```python
from build123d import *

# Parameters (mm, degrees)
SKETCH1_W           = 4.6
SKETCH1_H           = 4.6
BOSS_EXTRUDE1_DEPTH = 50


with BuildPart() as part:
    # Sketch1 → Boss-Extrude1 (new body, symmetric)
    with BuildSketch(Plane.XY):
        with BuildLine():
            Line((15, -13), (15, -4.4))
            ThreePointArc((15, -4.4), (14.853553391, -4.046446609), (14.5, -3.9))
            Line((14.5, -3.9), (13.5, -3.9))
            ThreePointArc((13.5, -3.9), (13.146446609, -4.046446609), (13, -4.4))
            Line((13, -4.4), (13, -6.6))
            ThreePointArc((13, -6.6), (12.853553391, -6.953553391), (12.5, -7.1))
            Line((12.5, -7.1), (8.297056275, -7.1))
            ThreePointArc((8.297056275, -7.1), (8.105714559, -7.061939766), (7.943502884, -6.953553391))
            Line((7.943502884, -6.953553391), (6.096446609, -5.106497116))
            ThreePointArc((6.096446609, -5.106497116), (5.988060234, -4.944285441), (5.95, -4.752943725))
            Line((5.95, -4.752943725), (5.95, 4.752943725))
            ThreePointArc((5.95, 4.752943725), (5.988060234, 4.944285441), (6.096446609, 5.106497116))
            Line((6.096446609, 5.106497116), (7.943502884, 6.953553391))
            ThreePointArc((7.943502884, 6.953553391), (8.105714559, 7.061939766), (8.297056275, 7.1))
            Line((8.297056275, 7.1), (12.5, 7.1))
            ThreePointArc((12.5, 7.1), (12.853553391, 6.953553391), (13, 6.6))
            Line((13, 6.6), (13, 4.4))
            ThreePointArc((13, 4.4), (13.146446609, 4.046446609), (13.5, 3.9))
            Line((13.5, 3.9), (14.5, 3.9))
            ThreePointArc((14.5, 3.9), (14.853553391, 4.046446609), (15, 4.4))
            Line((15, 4.4), (15, 13))
            ThreePointArc((15, 13), (14.414213562, 14.414213562), (13, 15))
            Line((13, 15), (4.4, 15))
            ThreePointArc((4.4, 15), (4.046446609, 14.853553391), (3.9, 14.5))
            Line((3.9, 14.5), (3.9, 13.5))
            ThreePointArc((3.9, 13.5), (4.046446609, 13.146446609), (4.4, 13))
            Line((4.4, 13), (6.6, 13))
            ThreePointArc((6.6, 13), (6.953553391, 12.853553391), (7.1, 12.5))
            Line((7.1, 12.5), (7.1, 8.297056275))
            ThreePointArc((7.1, 8.297056275), (7.061939766, 8.105714559), (6.953553391, 7.943502884))
            Line((6.953553391, 7.943502884), (5.106497116, 6.096446609))
            ThreePointArc((5.106497116, 6.096446609), (4.944285441, 5.988060234), (4.752943725, 5.95))
            Line((4.752943725, 5.95), (-4.752943725, 5.95))
            ThreePointArc((-4.752943725, 5.95), (-4.944285441, 5.988060234), (-5.106497116, 6.096446609))
            Line((-5.106497116, 6.096446609), (-6.953553391, 7.943502884))
            ThreePointArc((-6.953553391, 7.943502884), (-7.061939766, 8.105714559), (-7.1, 8.297056275))
            Line((-7.1, 8.297056275), (-7.1, 12.5))
            ThreePointArc((-7.1, 12.5), (-6.953553391, 12.853553391), (-6.6, 13))
            Line((-6.6, 13), (-4.4, 13))
            ThreePointArc((-4.4, 13), (-4.046446609, 13.146446609), (-3.9, 13.5))
            Line((-3.9, 13.5), (-3.9, 14.5))
            ThreePointArc((-3.9, 14.5), (-4.046446609, 14.853553391), (-4.4, 15))
            Line((-4.4, 15), (-13, 15))
            ThreePointArc((-13, 15), (-14.414213562, 14.414213562), (-15, 13))
            Line((-15, 13), (-15, 4.4))
            ThreePointArc((-15, 4.4), (-14.853553391, 4.046446609), (-14.5, 3.9))
            Line((-14.5, 3.9), (-13.5, 3.9))
            ThreePointArc((-13.5, 3.9), (-13.146446609, 4.046446609), (-13, 4.4))
            Line((-13, 4.4), (-13, 6.6))
            ThreePointArc((-13, 6.6), (-12.853553391, 6.953553391), (-12.5, 7.1))
            Line((-12.5, 7.1), (-8.297056275, 7.1))
            ThreePointArc((-8.297056275, 7.1), (-8.105714559, 7.061939766), (-7.943502884, 6.953553391))
            Line((-7.943502884, 6.953553391), (-6.096446609, 5.106497116))
            ThreePointArc((-6.096446609, 5.106497116), (-5.988060234, 4.944285441), (-5.95, 4.752943725))
            Line((-5.95, 4.752943725), (-5.95, -4.752943725))
            ThreePointArc((-5.95, -4.752943725), (-5.988060234, -4.944285441), (-6.096446609, -5.106497116))
            Line((-6.096446609, -5.106497116), (-7.943502884, -6.953553391))
            ThreePointArc((-7.943502884, -6.953553391), (-8.105714559, -7.061939766), (-8.297056275, -7.1))
            Line((-8.297056275, -7.1), (-12.5, -7.1))
            ThreePointArc((-12.5, -7.1), (-12.853553391, -6.953553391), (-13, -6.6))
            Line((-13, -6.6), (-13, -4.4))
            ThreePointArc((-13, -4.4), (-13.146446609, -4.046446609), (-13.5, -3.9))
            Line((-13.5, -3.9), (-14.5, -3.9))
            ThreePointArc((-14.5, -3.9), (-14.853553391, -4.046446609), (-15, -4.4))
            Line((-15, -4.4), (-15, -13))
            ThreePointArc((-15, -13), (-14.414213562, -14.414213562), (-13, -15))
            Line((-13, -15), (-4.4, -15))
            ThreePointArc((-4.4, -15), (-4.046446609, -14.853553391), (-3.9, -14.5))
            Line((-3.9, -14.5), (-3.9, -13.5))
            ThreePointArc((-3.9, -13.5), (-4.046446609, -13.146446609), (-4.4, -13))
            Line((-4.4, -13), (-6.6, -13))
            ThreePointArc((-6.6, -13), (-6.953553391, -12.853553391), (-7.1, -12.5))
            Line((-7.1, -12.5), (-7.1, -8.297056275))
            ThreePointArc((-7.1, -8.297056275), (-7.061939766, -8.105714559), (-6.953553391, -7.943502884))
            Line((-6.953553391, -7.943502884), (-5.106497116, -6.096446609))
            ThreePointArc((-5.106497116, -6.096446609), (-4.944285441, -5.988060234), (-4.752943725, -5.95))
            Line((-4.752943725, -5.95), (4.752943725, -5.95))
            ThreePointArc((4.752943725, -5.95), (4.944285441, -5.988060234), (5.106497116, -6.096446609))
            Line((5.106497116, -6.096446609), (6.953553391, -7.943502884))
            ThreePointArc((6.953553391, -7.943502884), (7.061939766, -8.105714559), (7.1, -8.297056275))
            Line((7.1, -8.297056275), (7.1, -12.5))
            ThreePointArc((7.1, -12.5), (6.953553391, -12.853553391), (6.6, -13))
            Line((6.6, -13), (4.4, -13))
            ThreePointArc((4.4, -13), (4.046446609, -13.146446609), (3.9, -13.5))
            Line((3.9, -13.5), (3.9, -14.5))
            ThreePointArc((3.9, -14.5), (4.046446609, -14.853553391), (4.4, -15))
            Line((4.4, -15), (13, -15))
            ThreePointArc((13, -15), (14.414213562, -14.414213562), (15, -13))
        make_face()
        with Locations((-11.1, -11.1)):
            Rectangle(SKETCH1_W, SKETCH1_H, mode=Mode.SUBTRACT)
        with Locations((11.1, -11.1)):
            Rectangle(SKETCH1_W, SKETCH1_H, mode=Mode.SUBTRACT)
        with Locations((11.1, 11.1)):
            Rectangle(SKETCH1_W, SKETCH1_H, mode=Mode.SUBTRACT)
        with BuildLine():
            Line((4.030508653, -2.828427125), (3.147361639, -1.945280111))
            ThreePointArc((3.147361639, -1.945280111), (3.7, 0), (3.147361639, 1.945280111))
            Line((3.147361639, 1.945280111), (4.030508653, 2.828427125))
            ThreePointArc((4.030508653, 2.828427125), (4.030508653, 4.030508653), (2.828427125, 4.030508653))
            Line((2.828427125, 4.030508653), (1.945280111, 3.147361639))
            ThreePointArc((1.945280111, 3.147361639), (0, 3.7), (-1.945280111, 3.147361639))
            Line((-1.945280111, 3.147361639), (-2.828427125, 4.030508653))
            ThreePointArc((-2.828427125, 4.030508653), (-4.030508653, 4.030508653), (-4.030508653, 2.828427125))
            Line((-4.030508653, 2.828427125), (-3.147361639, 1.945280111))
            ThreePointArc((-3.147361639, 1.945280111), (-3.7, 0), (-3.147361639, -1.945280111))
            Line((-3.147361639, -1.945280111), (-4.030508653, -2.828427125))
            ThreePointArc((-4.030508653, -2.828427125), (-4.030508653, -4.030508653), (-2.828427125, -4.030508653))
            Line((-2.828427125, -4.030508653), (-1.945280111, -3.147361639))
            ThreePointArc((-1.945280111, -3.147361639), (0, -3.7), (1.945280111, -3.147361639))
            Line((1.945280111, -3.147361639), (2.828427125, -4.030508653))
            ThreePointArc((2.828427125, -4.030508653), (4.030508653, -4.030508653), (4.030508653, -2.828427125))
        make_face(mode=Mode.SUBTRACT)
        with Locations((-11.1, 11.1)):
            Rectangle(SKETCH1_W, SKETCH1_H, mode=Mode.SUBTRACT)
    extrude(amount=BOSS_EXTRUDE1_DEPTH, both=True)


solid = part.part
```
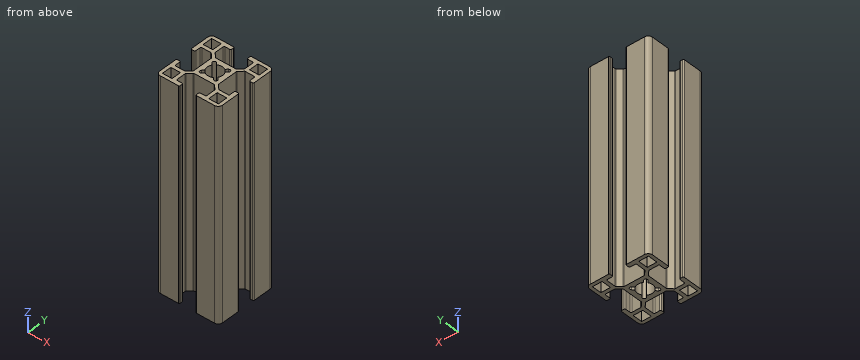
Build history of the part. All positions in model axes, mm. Give positions to 0.01 mm unless a question says otherwise; leave off trailing zeros. Loops run counter-clockwise (first coordinate to the right, second up) from the corner with the lowest first, then second, coordinate; pieces in that order, holes last.
Item 1: Drill centre lines: line 1 (Y direction, x = 11, z = 6.5); line 2 (X direction, y = -2.5, z = 19). Where is each one in solid material? Low to high.
Answers follow:
line 1: y = -15 to -13.4, -8.8 to -7.1, 7.1 to 8.8, 13.4 to 15
line 2: x = -5.95 to -3.7, 3.7 to 5.95
Item 2: Flat gauge pins, fed straight in: pin 1 (0.5 mm diameter, centred on x = 14, z = -5.5, fed in from -Y); pin 2 (3 mm diameter, centred on y = 0, z = -3.5, fed in from -X); pin 3 (0.8 mm diameter, centred on x = 14, z = -12, fed in from +Y). Where does each tip first touch, or does it go through?
Answers follow:
pin 1: stops at y = -14.85
pin 2: stops at x = -5.95
pin 3: stops at y = 14.91
Item 3: Slice it at B-B, the plane z = 36. Give the number of separate pieces and of enclosed holes in the cut face, and give its area (3 significant figures).
Answers follow:
separate pieces: 1
enclosed holes: 5
area: 311 mm2
Item 4: Slice it at A-A, the plane y = -0.75. List the corners of the cut face in (x, z).
Answers follow:
outline: (-5.95, -50) - (-3.62, -50) - (-3.62, 50) - (-5.95, 50) - close; (3.62, -50) - (5.95, -50) - (5.95, 50) - (3.62, 50) - close
